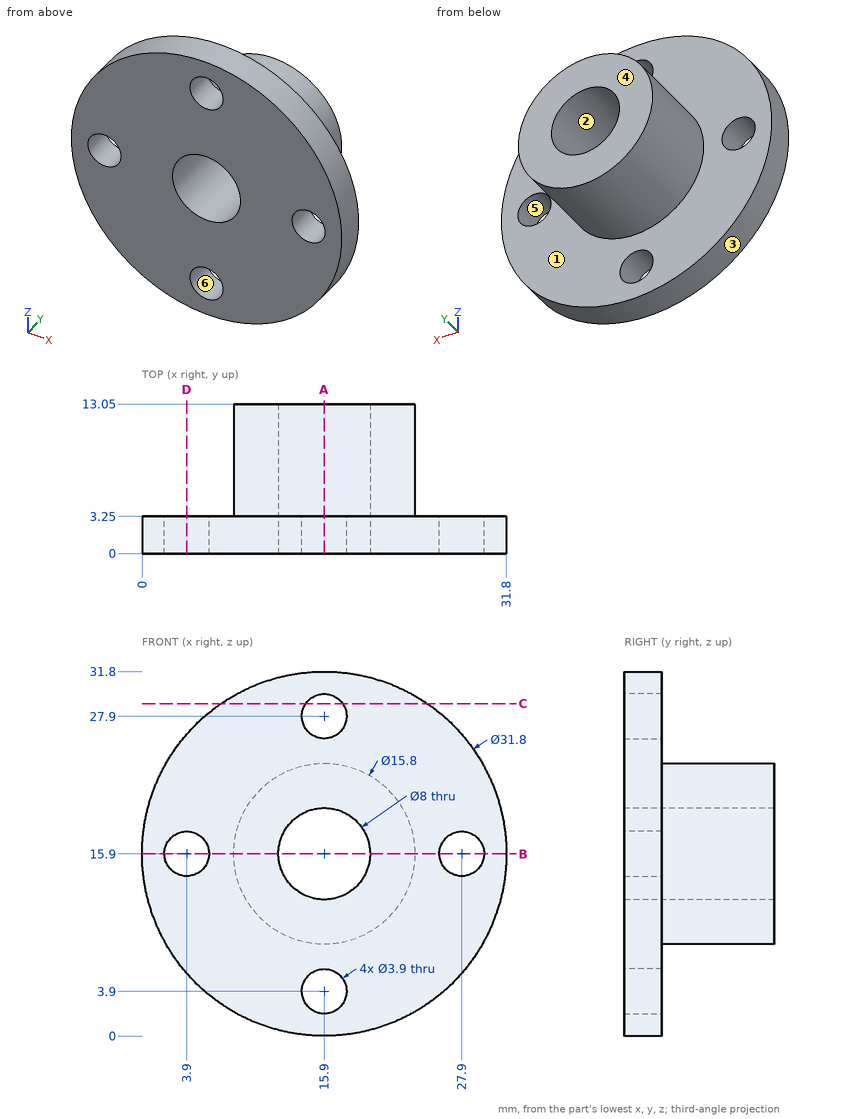
Job drawing, mm, ordinate dimensions from the low corner. One solid piece. A direction names the side the tool comes from. Round coordinates to 2 decimals unless told otherwise and drop trailing zeros. Write each loop counter-clockwise with the first axis right and the second up, starting at its lowest first coordinate (ties: lowest second). Pieces come first, ordered by that corner, then holes.
1) 3-axis set-ups, long thin cutter, end or side, ignore diameter. For the marked faces 1 and 2: which of +Z, -Z, +X, -X, +Y, -Y reach the whole face in a straight line?
2) Band-saw the part on D-D, the plane x = 3.9. List the corners of the cut face in (y, z).
3) Pin check, flat tips, straight feed: pin 1 (3 mm diameter, centred on x = 15.9, z = 27.9, fed in from +Y); pin 2 (2 mm diameter, centred on y = 8, z = 22, fed in from -X); pin 3 (4 mm diameter, centred on x = 24.5, y = 10.5, fed in from +Z); pin 4 (2 mm diameter, centred on x = 6.5, z = 17.5, fed in from +Y). Stop position of each tip, or through.
4) Band-saw the part on A-A, the plane x = 15.9. List the corners of the cut face in (y, z).
5) Band-saw the part on B-B, the plane z = 15.9. List the corners of the cut face in (x, y), and give its area (3 significant figures).
6) Mould opens along X. For the marked faces 3, 4, 5 and 6 say: +X half, -X half, draft (parallel to the pull), parting line (faces both ways), or undercut.
7) Drill centre lines: probe 1 along X at (y, z) = (1.65, 15.9); probe 2 along X at (y, z) = (5.75, 15.9); probe 3 along Y at (x, z) = (1.5, 10.5). Where is each one in solid material? Low to high.
8) Band-saw the part on C-C, the plane z = 29. List the corners of the cut face in (x, y).
Ans:
1. face 1: +Y
1. face 2: +Y, -Y
2. outline: (0, 5.47) - (3.25, 5.47) - (3.25, 13.95) - (0, 13.95) - close; (0, 17.85) - (3.25, 17.85) - (3.25, 26.33) - (0, 26.33) - close
3. pin 1: passes through
3. pin 2: stops at x = 9.87
3. pin 3: stops at z = 20.24
3. pin 4: stops at y = 3.25
4. outline: (0, 0) - (3.25, 0) - (3.25, 1.95) - (0, 1.95) - close; (0, 5.85) - (3.25, 5.85) - (3.25, 8) - (13.05, 8) - (13.05, 11.9) - (0, 11.9) - close; (0, 19.9) - (13.05, 19.9) - (13.05, 23.8) - (3.25, 23.8) - (3.25, 25.95) - (0, 25.95) - close; (0, 29.85) - (3.25, 29.85) - (3.25, 31.8) - (0, 31.8) - close
5. outline: (0, 0) - (1.95, 0) - (1.95, 3.25) - (0, 3.25) - close; (5.85, 0) - (11.9, 0) - (11.9, 13.05) - (8, 13.05) - (8, 3.25) - (5.85, 3.25) - close; (19.9, 0) - (25.95, 0) - (25.95, 3.25) - (23.8, 3.25) - (23.8, 13.05) - (19.9, 13.05) - close; (29.85, 0) - (31.8, 0) - (31.8, 3.25) - (29.85, 3.25) - close
5. area: 128 mm2
6. face 3: parting line
6. face 4: draft
6. face 5: undercut
6. face 6: undercut
7. probe 1: x = 0 to 1.95, 5.85 to 11.9, 19.9 to 25.95, 29.85 to 31.8
7. probe 2: x = 8 to 11.9, 19.9 to 23.8
7. probe 3: y = 0 to 3.25
8. outline: (6.89, 0) - (14.29, 0) - (14.29, 3.25) - (6.89, 3.25) - close; (17.51, 0) - (24.91, 0) - (24.91, 3.25) - (17.51, 3.25) - close
